from build123d import *

# Parameters (mm, degrees)
F1_DEPTH = 9
F2_W     = 325
F2_H     = 265
F2_R     = 13
F3_DEPTH = 25


with BuildPart() as f1:
    # F0 (on Top) → F1 (new body)
    with BuildSketch(Plane.XY):
        Polygon((410, 0), (410, 841), (295, 841), (295, 363), (0, 363), (0, 0), align=None)
    extrude(amount=F1_DEPTH)

    # F2 (on face) → F3 (cut)
    with BuildSketch(Plane.XY.offset(9)):
        with Locations((217.5, 181.5)):
            Rectangle(F2_W, F2_H)
        with Locations((27.5, 314)):
            Circle(F2_R)
    extrude(amount=-F3_DEPTH, mode=Mode.SUBTRACT)


solid = f1.part
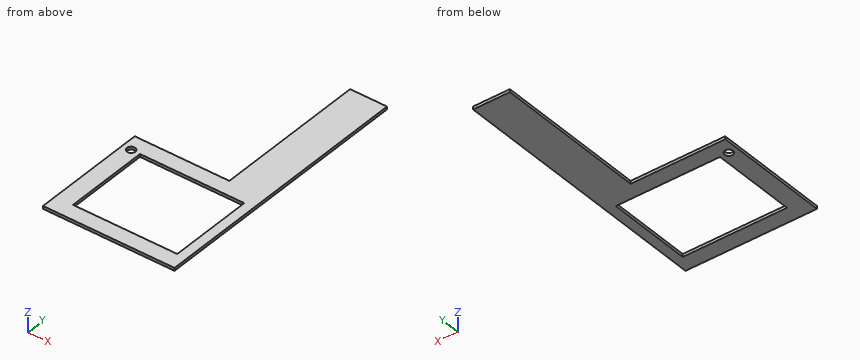
Input: part model. Units: mm. Frame: model coordinates. Give positions to 0.01 mm unless a question says otherwise; leave off trailing zeros. Write each loop counter-clockwise with the first axis right and the second up, starting at its lowest first coordinate (ties: lowest second). Pieces come first, ordered by that corner, then holes.
Q1. Material intervals for probe 1 along Y at (x, z) = (113, 6.75); probe 2 along Y at (x, z) = (27.5, 3.5); probe 3 along X at (y, z) = (100, 4), sorted ascending.
Q2. Section C-C, the plane y = 783.5. Output: boundary loops of the cut face in (x, z).
Q3. Section B-B, the plane x = 343. Output: boundary loops of the cut face in (y, z), plus the area to 3 significant figures.
Q4. Section A-A, the plane x = 283. Output: boundary loops of the cut face in (y, z), plus the area to 3 significant figures.
Q5. First-contact query: P1, Ø4, axis at y = 570, z = 1.5, coming from the -X side; P2, Ø21, axis at x = 27.5, y = 314, coming from the -Z side; P3, Ø2.5, axis at x = 113.5, z = 5, coming from the +Y side; P4, Ø4.5, axis at x = 239.5, z = 3, coming from the -Y side. Flat tips, straight axial feed; report the tip coordinate or a pass-through.
Filled in:
1. probe 1: y = 0 to 49, 314 to 363
1. probe 2: y = 0 to 301, 327 to 363
1. probe 3: x = 0 to 55, 380 to 410
2. outline: (295, 0) - (410, 0) - (410, 9) - (295, 9) - close
3. outline: (0, 0) - (49, 0) - (49, 9) - (0, 9) - close; (314, 0) - (841, 0) - (841, 9) - (314, 9) - close
3. area: 5,180 mm2
4. outline: (0, 0) - (49, 0) - (49, 9) - (0, 9) - close; (314, 0) - (363, 0) - (363, 9) - (314, 9) - close
4. area: 882 mm2
5. P1: stops at x = 295
5. P2: passes through
5. P3: stops at y = 363
5. P4: stops at y = 0
